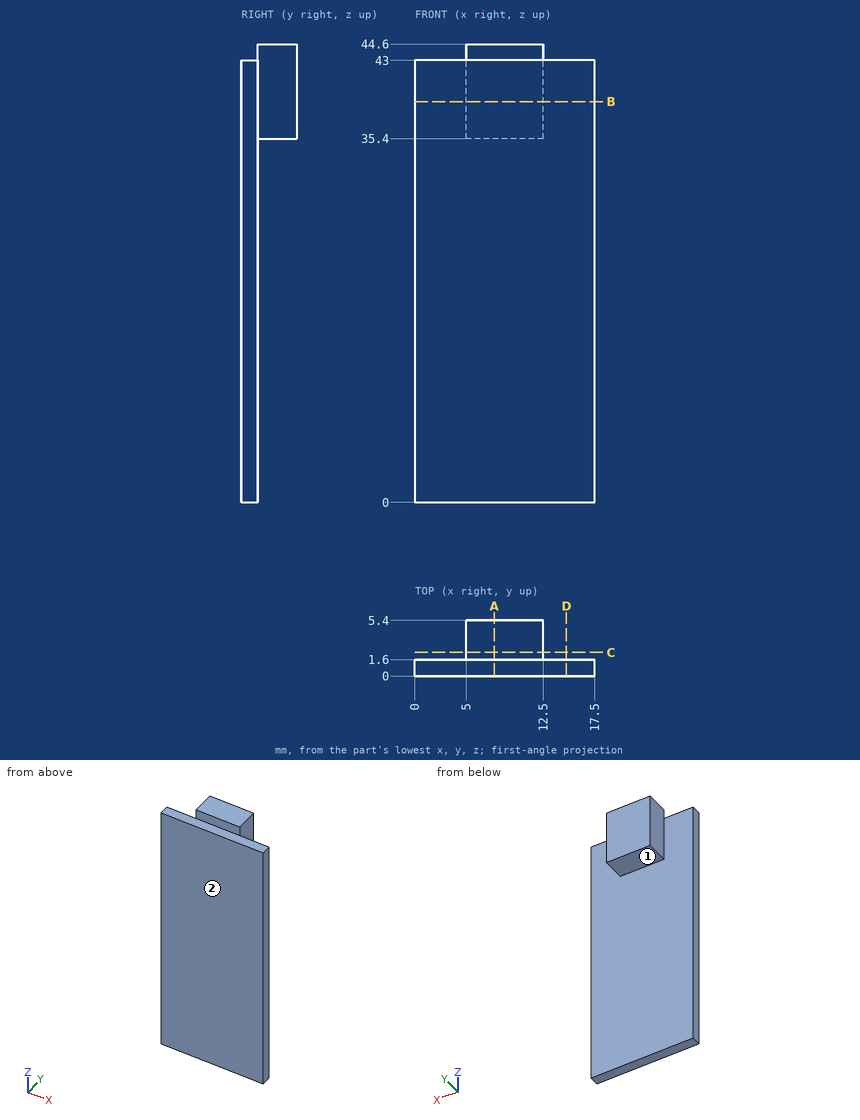
Study the drawing (mm; zero at the part's minimum x, y, z) and answer. A direction names the side the tool comes from. Give positions to 0.01 mm unless a question says otherwise; leave off trailing zeros. Loops run counter-clockwise (first coordinate to the right, second up) from the corner with the lowest first, then second, coordinate; pieces in that order, holes last. Notation, with made-up numbers: (-23.75, 69.5) - (-12.75, 69.5) arc R24 ccw to (-12.75, 101.5) - close; hole circle Ø3 at (-4, -28). An arc over 180 degrees is marked (long way). Use CSV: the item, a comma, the result in double quotes. Start each with the question number.
(1) Find section B-B, the plane z = 39. Determine the outline of the cut face in (x, y), plus the area to 3 significant figures.
(2) Find section D-D, the plane x = 14.75. Determine the outline of the cut face in (y, z), plus the area to 3 significant figures.
(3) Find section C-C, the plane y = 2.3. Determine the outline of the cut face in (x, z), plus the area to 3 significant figures.
(4) Find the intervals of material crossed by L1, parallel to Z at x = 6, y = 5.15; L2, parallel to Y at x = 2.5, z = 15; L3, parallel to X at y = 2.7, z = 37, in increasing order.
(5) Each of these flat-tipped pins is pushed along its axis until it touches: pin 1 (1.1 mm diameter, centred on x = 9.5, y = 3, fed in from -Z); pin 2 (2 mm diameter, centred on x = 12, z = 13.5, fed in from +Y); pin 3 (1.1 mm diameter, centred on y = 4, z = 40.5, fed in from -X). Where does it stop, or does it pass through?
(6) A tool of negligible diameter and unlimited length cuts with its end or side. For the marked faces 1 and 2, from which of +Z, -Z, +X, -X, +Y, -Y can it reach the whole face along a straight path? Write none if from no direction.
(7) Find section A-A, the plane x = 7.75. Determine the outline of the cut face in (y, z).
Results found:
1,outline,"(0, 0) - (17.5, 0) - (17.5, 1.6) - (12.5, 1.6) - (12.5, 5.4) - (5, 5.4) - (5, 1.6) - (0, 1.6) - close"
1,area,"56.5 mm^2"
2,outline,"(0, 0) - (1.6, 0) - (1.6, 43) - (0, 43) - close"
2,area,"68.8 mm^2"
3,outline,"(5, 35.4) - (12.5, 35.4) - (12.5, 44.6) - (5, 44.6) - close"
3,area,"69.0 mm^2"
4,L1,"35.4 to 44.6"
4,L2,"0 to 1.6"
4,L3,"5 to 12.5"
5,pin 1,"z = 35.4"
5,pin 2,"y = 1.6"
5,pin 3,"x = 5"
6,face 1,"-Z, +X, -X, +Y"
6,face 2,"+Z, -Z, +X, -X, -Y"
7,outline,"(0, 0) - (1.6, 0) - (1.6, 35.4) - (5.4, 35.4) - (5.4, 44.6) - (1.6, 44.6) - (1.6, 43) - (0, 43) - close"
